```python
from build123d import *

# Parameters (mm, degrees)
F2_R     = 4.5
F3_R     = 12.65
F4_DEPTH = 35.001
F5_SIZE  = 0.75


with BuildPart() as f1:
    # F0 (on Front) → F1 (revolve)
    with BuildSketch(Plane.XZ):
        Polygon((-17.5, 0), (0, 0), (17.5, 0), (17.5, 18), (6.5, 18), (6.5, 24.25), (-6.5, 24.25), (-6.5, 18), (-17.5, 18), align=None)
    revolve(axis=Axis((-8.75, 0, 0), (-1, 0, 0)))

    # F2
    f2_edges = [f1.edges().sort_by_distance(p)[0] for p in [
        (6.5, 0, -18),
        (-6.5, 0, -18),
    ]]
    fillet(f2_edges, radius=F2_R)

    # F3 (on face) → F4 (cut, through all)
    with BuildSketch(Plane.YZ.offset(17.5)):
        Circle(F3_R)
    extrude(amount=-F4_DEPTH, mode=Mode.SUBTRACT)

    # F5
    f5_edges = [f1.edges().sort_by_distance(p)[0] for p in [
        (17.5, -12.65, 0),
        (0, 12.65, 0),
        (-17.5, -12.65, 0),
        (-6.5, 0, -24.25),
        (-17.5, 0, -18),
        (6.5, 0, -24.25),
        (17.5, 0, -18),
    ]]
    chamfer(f5_edges, length=F5_SIZE)


solid = f1.part
```
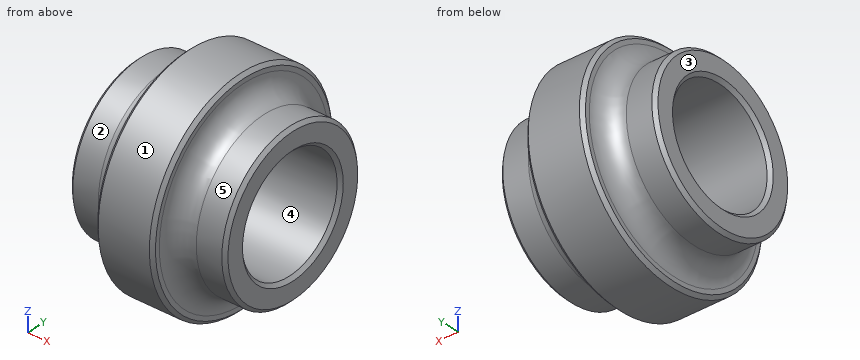
The model under review builds one solid part; all positions refer to its coordinate system, in mm. Face numbers are marked on the shaded views. A direction names the side the tool comes from. Round coordinates to 2 decimals unless told otherwise and drop trailing zeros. Loops run counter-clockwise (first coordinate to the right, second up) from the corner with the lowest first, then second, coordinate; pieces in that order, holes last. Notation, with made-up numbers: M 31.5,64 L 81.5,64 A5 ccw 81.5,68 Z; hole C -37,-10.5 d7. An arc over 180 degrees is marked long. Write item = value, one per line.
Item 1: For line 1 (Y direction, x = -16, z = -4); line 2 (Y direction, x = 6, z = -3); line 3 (Z direction, x = 1, y = 2.5), list the stretches that pass through material, from the lowest coordinate up. Write a range as [from, to].
Return value:
line_1 = [-17.55, -12], [12, 17.55]
line_2 = [-23.81, -12.29], [12.29, 23.81]
line_3 = [-24.12, -12.4], [12.4, 24.12]
Item 2: Take a section at C-C on x = 15.5. Write out the cut boundary in (y, z), then the cut area to 3 significant figures.
Return value:
outline = C 0,0 d36; hole C 0,0 d25.3
area = 515 mm2
Item 3: The part is to be moulded in two halves that separate along Y. For the marked faces 3, 4 and 5, say which applies: released by +Y, released by -Y, zero draft, split by the parting line, or undercut.
Return value:
face_3 = zero draft
face_4 = undercut
face_5 = split by the parting line
Item 4: Machinability: for the marked faces 1 and 2, which of the approach directions +Z, -Z, +X, -X, +Y, -Y give a long, thin tool a straight path to every point of the face, cutting with its end or side? Answer none if there is none.
Return value:
face_1 = +X, -X
face_2 = -X
Item 5: Insertion check: P1, Ø1.5, axis at x = 13.5, y = 19, coming from the +Z side; P2, Ø2, axis at x = 9.5, z = -9, coming from the +Y side; P3, Ø4, axis at x = -3.5, y = 10, coming from the -Z side. Each pin has a flat end and moves straight along its axis. Give the tip position at first contact, or say it passes through.
Return value:
P1 = through
P2 = 16.63
P3 = -22.89
Item 6: Take a section at D-D on x = 2.5. Write out the cut boundary in (y, z), then the cut area to 3 significant figures.
Return value:
outline = C 0,0 d48.5; hole C 0,0 d25.3
area = 1,340 mm2
